from build123d import *

# Parameters (mm, degrees)
BOSS_EXTRUDE1_DEPTH       = 200
CUT_EXTRUDE1_DEPTH        = 250.198715888
F_6_0MM_DOWEL_SLOT1_DEPTH = 20
M6X1_0_TAPPED_HOLE1_D     = 5
M6X1_0_TAPPED_HOLE1_DEPTH = 21.497848452
M6X1_0_TAPPED_HOLE1_TIP   = 1.502151548
FILLET1_R                 = 6
FILLET2_R                 = 20


# Read off the part's stored shape, not the designer's step: Ø6.0mm Dowel Slot1
with BuildPart() as part:
    # Sketch1 → Boss-Extrude1 (new body)
    with BuildSketch(Plane.XY):
        Polygon((-21, 207), (-148, 207), (-148, 197.5), (-148, 193), (-24, 193), (-12, 193), (-12, 207), align=None)
    extrude(amount=BOSS_EXTRUDE1_DEPTH)

    # Sketch3 → Cut-Extrude1 (cut, through all)
    with BuildSketch(Plane(origin=(0, 207, 0), x_dir=(1, 0, 0), z_dir=(0, 1, 0))):
        Polygon((-128, -20), (-128, -30), (-128, -108), (-128, -180), (-118, -180), (-54, -180), (-32, -180), (-32, -20), align=None)
    extrude(amount=-CUT_EXTRUDE1_DEPTH, mode=Mode.SUBTRACT)

    # Ø6.0mm Dowel Slot1 outline → Ø6.0mm Dowel Slot1 (cut)
    with BuildSketch(Plane.XY):
        with BuildLine():
            Line((-52.5, 196.5), (-47.5, 196.5))
            ThreePointArc((-47.5, 196.5), (-44, 200), (-47.5, 203.5))
            Line((-47.5, 203.5), (-52.5, 203.5))
            ThreePointArc((-52.5, 203.5), (-56, 200), (-52.5, 196.5))
        make_face()
        with BuildLine():
            ThreePointArc((-77.5, 196.5), (-74, 200), (-77.5, 203.5))
            Line((-77.5, 203.5), (-82.5, 203.5))
            ThreePointArc((-82.5, 203.5), (-86, 200), (-82.5, 196.5))
            Line((-82.5, 196.5), (-77.5, 196.5))
        make_face()
        with BuildLine():
            ThreePointArc((-107.5, 196.5), (-104, 200), (-107.5, 203.5))
            Line((-107.5, 203.5), (-112.5, 203.5))
            ThreePointArc((-112.5, 203.5), (-116, 200), (-112.5, 196.5))
            Line((-112.5, 196.5), (-107.5, 196.5))
        make_face()
    extrude(amount=F_6_0MM_DOWEL_SLOT1_DEPTH, mode=Mode.SUBTRACT)

    # M6x1.0 Tapped Hole1
    with Locations(Plane.XY.offset(200)):
        with Locations((-119, 200), (-54, 200)):
            Hole(M6X1_0_TAPPED_HOLE1_D / 2, depth=M6X1_0_TAPPED_HOLE1_DEPTH)
            with Locations((0, 0, -(M6X1_0_TAPPED_HOLE1_DEPTH + M6X1_0_TAPPED_HOLE1_TIP / 2))):  # 118° drill point
                Cone(0, M6X1_0_TAPPED_HOLE1_D / 2, M6X1_0_TAPPED_HOLE1_TIP, mode=Mode.SUBTRACT)

    # Fillet1
    fillet1_edges = [part.edges().sort_by_distance(p)[0] for p in [
        (-128, 200, 180),
        (-128, 200, 20),
        (-32, 200, 20),
    ]]
    fillet(fillet1_edges, radius=FILLET1_R)

    # Fillet2
    fillet2_edges = [part.edges().sort_by_distance(p)[0] for p in [
        (-12, 200, 200),
        (-32, 200, 180),
    ]]
    fillet(fillet2_edges, radius=FILLET2_R)


solid = part.part
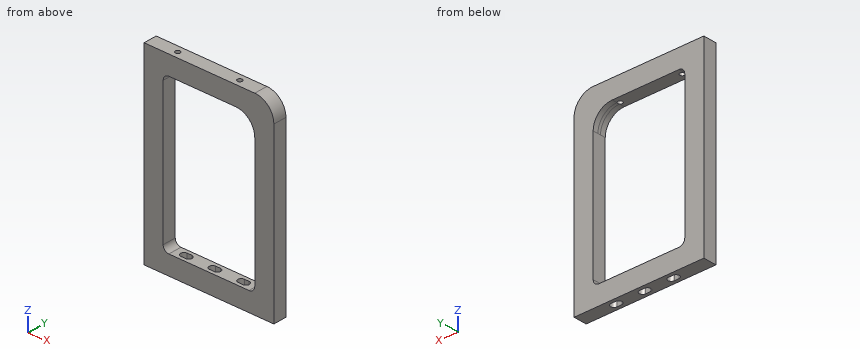
Work out the finished part from the listing and answer in its coordinate system (mm). Coordinates: 2 decimals unless noted, no trailing zeros. Order: outer loops, then holes, each group sorted by start corner. A loop starts at its lowest first (then second) coordinate and runs counter-clockwise, first axis right, second up. Notation, with made-up numbers: (47.5, -36.75) - (64.5, -36.75) arc R18 ccw to (64.5, -16.75) - close; hole circle Ø8 at (-2.75, -20). An arc over 180 degrees is marked (long way). Put each result on its own line as item: value. Start each with the question number.
1) Find section A-A (x = -100). Give the vertices of the cut face in (y, z), plus the area to 3 significant figures.
2) Find the intervals of material crossed by line 1 (Y direction, x = -54, z = 188); line 2 (X direction, y = 197.5, z = 18); line 3 (X direction, y = 205, z = 120), in increasing order. Write a range as from..to.
3) Flat-ended cylindrical pins translate along their axes: pin 1 (1 mm diameter, centred on x = -123.5, y = 205, fed in from -Z); pin 2 (4.5 mm diameter, centred on x = -54, y = 200, fed in from +Z). Find the tip coordinate at first contact, or state that the pin passes through.
4) Find section B-B (z = 152). Give the vertices of the cut face in (x, y), plus the area to 3 significant figures.
Results list:
1. outline: (193, 0) - (207, 0) - (207, 20) - (193, 20) - close; (193, 180) - (207, 180) - (207, 200) - (193, 200) - close
1. area: 560 mm^2
2. line 1: y = 193..197.5, 202.5..207
2. line 2: x = -148..-114.95, -105.05..-84.95, -75.05..-54.95, -45.05..-12
2. line 3: x = -148..-128, -32..-12
3. pin 1: stops at z = 0
3. pin 2: stops at z = 20
4. outline: (-148, 193) - (-128, 193) - (-128, 207) - (-148, 207) - close; (-32, 193) - (-12, 193) - (-12, 207) - (-32, 207) - close
4. area: 560 mm^2
